Geometry check sheet. Reference: the model listing, model coordinates, mm. A direction names the side the tool comes from. Give positions to 0.01 mm unless a question says otherwise; leave off trailing zeros. Write each loop counter-clockwise with the first axis right and the second up, starting at its lowest first coordinate (ties: lowest second). Pieces come first, ordered by that corner, then holes. Notation, with made-up numbers: M -22.75,27.5 L 1.25,27.5 A5 cw 1.25,34.5 Z; hole C 80.5,29 d9. An arc over 180 degrees is marked long. One line per item, written item: value. Start each with the question number.
1. Scan lines: line 1 (X direction, y = 6.5, z = 14.5); line 2 (Z direction, x = -5, y = -47); line 3 (Z direction, x = 2.5, y = -8.5). Record each from-to range of solid material in increasing order.
2. Tool access check on faces 4 (the face through (-13.72, 30.67, 17.37)), 5 (the face through (13.72, 9.33, 17.37)), 6 (the face through (2.285, 3.584, 17.366)). Record the directions out of +Z, -Z, +X, -X, +Y, -Y that give a thin tool (end or side, any length) a straight path to the whole face; none if there is none.
3. Release check for a two-part mould opening along X. For faces 1 (the face through (-13.78, 9.17, 17.37)), 2 (the face through (-31.1, -6, 8)), 3 (the face through (0, -76, 8)) record: pulls with the +X half, pulls with the -X half, needs draft (parallel to the pull), parting line crosses it, or undercut.
4. Cross-section at C-C on y = 40. Record the cut outline in (x, z).
5. Cross-section at A-A on y = -22.5. Record the cut outline in (x, z), then the cut area to 3 significant figures.
6. Gauge pin test, flat ends, axial feed: pin 1 (1 mm diameter, centred on x = 3.5, z = 15, fed in from -Y); pin 2 (0.6 mm diameter, centred on y = -28.5, z = 16, fed in from +X); pin 3 (2 mm diameter, centred on x = 15.5, z = 17, fed in from -Y). Record the tip position at first contact, or that the pin passes through.
from build123d import *

# Parameters (mm, degrees)
F0_W     = 62.2
F0_H     = 152
F1_DEPTH = 16.38
F2_R     = 20
F3_R     = 31.09999
F4_R     = 2
F5_W     = 37.4
F5_H     = 40.62
F6_DEPTH = 2
F7_R     = 4.25
F8_DEPTH = 2


# Not quite as in the source:
# - a fillet or chamfer is up to 0.001 mm smaller than in the source, because OpenCascade refuses the exact size


with BuildPart() as f1:
    # F0 (on Top) → F1 (new body)
    with BuildSketch(Plane.XY):
        Rectangle(F0_W, F0_H)
    extrude(amount=F1_DEPTH)

    # F2
    f2_edges = [f1.edges().sort_by_distance(p)[0] for p in [
        (-31.1, -76, 8.19),
        (31.1, -76, 8.19),
    ]]
    fillet(f2_edges, radius=F2_R)

    # F3 (radius 31.1 in the source; OpenCascade refuses exactly that, so slightly less here)
    f3_edges = [f1.edges().sort_by_distance(p)[0] for p in [
        (31.1, 76, 8.19),
        (-31.1, 76, 8.19),
    ]]
    fillet(f3_edges, radius=F3_R)

    # F4
    f4_edges = [f1.edges().sort_by_distance(p)[0] for p in [
        (31.1, -5.549995, 16.38),
        (31.1, -5.549995, 0),
    ]]
    fillet(f4_edges, radius=F4_R)

    # F5 (on face) → F6 (cut)
    with BuildSketch(Plane.XY.offset(16.38)):
        with Locations((0, -35.31)):
            Rectangle(F5_W, F5_H)
    extrude(amount=-F6_DEPTH, mode=Mode.SUBTRACT)

    # F7 (on face) → F8 (join)
    with BuildSketch(Plane.XY.offset(16.38)):
        Polygon((11.5, 15), (16, 3.5), (20.5, 15), align=None)
        Circle(F7_R)
        Polygon((-16, 3.5), (-11.5, 15), (-20.5, 15), align=None)
        Polygon((-20.5, 25), (-11.5, 25), (-16, 36.5), align=None)
        with Locations((0, 20)):
            Circle(F7_R)
        Polygon((11.5, 25), (20.5, 25), (16, 36.5), align=None)
        with Locations((0, 40)):
            Circle(F7_R)
    extrude(amount=F8_DEPTH)


solid = f1.part
Report:
1. line 1: x = -31.1 to 31.1
1. line 2: z = 0 to 14.38
1. line 3: z = 0 to 16.38
2. face 4: +Z, +Y
2. face 5: +Z, -Y
2. face 6: +Z
3. face 1: undercut
3. face 2: pulls with the -X half
3. face 3: needs draft
4. outline: M -31.1,2 A2 ccw -29.1,0 L 29.1,0 A2 ccw 31.1,2 L 31.1,14.38 A2 ccw 29.1,16.38 L 4.25,16.38 L 4.25,18.38 L -4.25,18.38 L -4.25,16.38 L -29.1,16.38 A2 ccw -31.1,14.38 Z
5. outline: M -31.1,2 A2 ccw -29.1,0 L 29.1,0 A2 ccw 31.1,2 L 31.1,14.38 A2 ccw 29.1,16.38 L 18.7,16.38 L 18.7,14.38 L -18.7,14.38 L -18.7,16.38 L -29.1,16.38 A2 ccw -31.1,14.38 Z
5. area: 941 mm^2
6. pin 1: stops at y = -76
6. pin 2: stops at x = 30.6
6. pin 3: stops at y = -74.68
